```python
from build123d import *

# Parameters (mm, degrees)
SKETCH2_W           = 8
SKETCH2_H           = 9.6
SKETCH4_R           = 2.4
BOSS_EXTRUDE1_DEPTH = 1.6
LPATTERN1_COUNT     = 2
LPATTERN1_PITCH     = 8
SKETCH5_R           = 2.4
BOSS_EXTRUDE2_DEPTH = 1.6
LPATTERN2_COUNT     = 2
LPATTERN2_PITCH     = 8
SHELL1_T            = -1.6


with BuildPart() as part:
    # Sweep1: sweep along a path in Sketch3
    with BuildLine(Plane.XY) as sweep1_path:
        Line((0, 0), (20, 0))
        Line((20, 0), (39.318516526, 5.176380902))
    # Sketch2 → Sweep1 (sweep)
    with BuildSketch(Plane(origin=(0, 0, 0), x_dir=(0, 0, -1), z_dir=(1, 0, 0))):
        Rectangle(SKETCH2_W, SKETCH2_H)
    sweep(path=sweep1_path.line, transition=Transition.RIGHT)

    # Sketch4 → Boss-Extrude1 (add)
    with BuildSketch(Plane(origin=(0, 4.8, 0), x_dir=(1, 0, 0), z_dir=(0, 1, 0))):
        with Locations(Location((4, 0, 0), (0, 0, 270))):
            Circle(SKETCH4_R)
    boss_extrude1 = extrude(amount=BOSS_EXTRUDE1_DEPTH)

    # LPattern1: Boss-Extrude1 ×2
    with Locations(*[(i * LPATTERN1_PITCH, 0, 0) for i in range(1, LPATTERN1_COUNT)]):
        add(boss_extrude1)

    # Sketch5 → Boss-Extrude2 (add)
    with BuildSketch(Plane(origin=(0.097414546, -0.363556034, 0), x_dir=(0.9659258262890681, 0.2588190451025216, 0), z_dir=(-0.2588190451025216, 0.9659258262890681, 0))):
        with Locations(Location((35.318516526, 0, 0), (0, 0, 180))):
            Circle(SKETCH5_R)
    boss_extrude2 = extrude(amount=BOSS_EXTRUDE2_DEPTH)

    # LPattern2: Boss-Extrude2 ×2
    with Locations(*[Vector(-0.9659258262890681, -0.2588190451025219, 0) * (i * LPATTERN2_PITCH) for i in range(1, LPATTERN2_COUNT)]):
        add(boss_extrude2)

    # Shell1
    shell1_openings = [part.faces().sort_by_distance(p)[0] for p in [
        (10.315965994, -4.8, 0),
        (30.596389965, -2.130031532, 0),
    ]]
    offset(amount=SHELL1_T, openings=shell1_openings, kind=Kind.INTERSECTION)


solid = part.part
```
Here's how the part is built. I have some questions about the finished solid (model axes, mm). A direction names the side the tool comes from. Give positions to 0.01 mm unless a question says otherwise; leave off trailing zeros. Order: outer loops, then holes, each group sorted by start corner. A loop starts at its lowest first (then second) coordinate and runs counter-clockwise, first axis right, second up. Notation, with made-up numbers: (50.25, -15) -> (94.25, -15) arc R30 cw to (94.25, 7) -> close; hole circle Ø3 at (29.5, -8). An arc over 180 degrees is marked (long way). Use CSV: the item, a comma, the result in double quotes. Start each with the question number.
Item 1: If I drill on probe 1 along Z at (x, y) = (12, 3.95); probe 2 along Z at (x, y) = (8.5, -2); probe 3 along Y at (x, z) = (14, -0.75), over which ranges is the centre line in solid material (lowest first)? Write a range as [from, to].
Item 2: Suppose I cut it at D-D (y = -2). List the corners of the cut face in (x, z) for me.
Item 3: I'm going to push flat-ended pins straight in: P1, Ø3, axis at y = 1.5, z = 1.5, coming from the -X side; P2, Ø1.3, axis at x = 12, z = 0, coming from the +Y side; P3, Ø0.8, axis at x = 4, z = 0, coming from the -Y side; P4, Ø2, axis at x = 4, z = 0, coming from the -Y side. Where does each tip first touch, or does it pass through?
Item 4: Suppose I cut it at B-B (y = 5.5). Give the number of separate pieces and of enclosed holes in the cut face, and give its area (3 significant figures).
Item 5: Suppose I cut it at C-C (z = 3.25). List the corners of the cut face in (x, y) for me.
Item 6: Suppose I cut it at A-A (x = 12). List the corners of the cut face in (y, z) for me, and give its area (3 significant figures).
Item 7: On a 3-axis mill with a long thin cutter (end or side, diameter ignored), from which of +Z, -Z, +X, -X, +Y, -Y can I reach the whole of each face in a straight line? I mean faces 4 (the cylindrical face through (3.22, 3.99, -0.17)), 5 (the flat face through (10, 4.8, -2)), 6 (the flat face through (4, 6.4, 0)), 7 (the flat face through (34.22, 8.78, 0.01)). Say none if no direction works.
Item 8: Thinking about a two-plate mould opening in Z: for faces 1 (the flat face through (11, 3.2, 0)), 2 (the flat face through (21, 1, 4)), 3 (the cylindrical face through (14.38, 5.59, -0.31)), which applies, pulls with the +Z half, pulls with the -Z half, needs draft (parallel to the pull), parting line crosses it, or undercut?
Answer block:
1,probe 1,"z = [-4, -0.8], [0.8, 4]"
1,probe 2,"z = [-4, -2.4], [2.4, 4]"
1,probe 3,"y = [3.2, 6.4]"
2,outline,"(0, -4) -> (31.08, -4) -> (31.08, -2.4) -> (1.6, -2.4) -> (1.6, 2.4) -> (31.08, 2.4) -> (31.08, 4) -> (0, 4) -> close"
3,P1,"stops at x = 0"
3,P2,"stops at y = 6.4"
3,P3,"stops at y = 4.8"
3,P4,"stops at y = 3.2"
4,separate pieces,"3"
4,enclosed holes,"2"
4,area,"127 mm^2"
5,outline,"(0, -4.8) -> (20.63, -4.8) -> (40.56, 0.54) -> (38.08, 9.81) -> (19.37, 4.8) -> (0, 4.8) -> close"
6,outline,"(-4.8, -4) -> (4.8, -4) -> (4.8, -2.4) -> (6.4, -2.4) -> (6.4, 2.4) -> (4.8, 2.4) -> (4.8, 4) -> (-4.8, 4) -> (-4.8, 2.4) -> (3.2, 2.4) -> (3.2, 0.8) -> (4.8, 0.8) -> (4.8, -0.8) -> (3.2, -0.8) -> (3.2, -2.4) -> (-4.8, -2.4) -> close"
6,area,"43.5 mm^2"
7,face 4,"-Y"
7,face 5,"+Y"
7,face 6,"+Z, -Z, -X, +Y"
7,face 7,"none"
8,face 1,"undercut"
8,face 2,"pulls with the +Z half"
8,face 3,"parting line crosses it"
